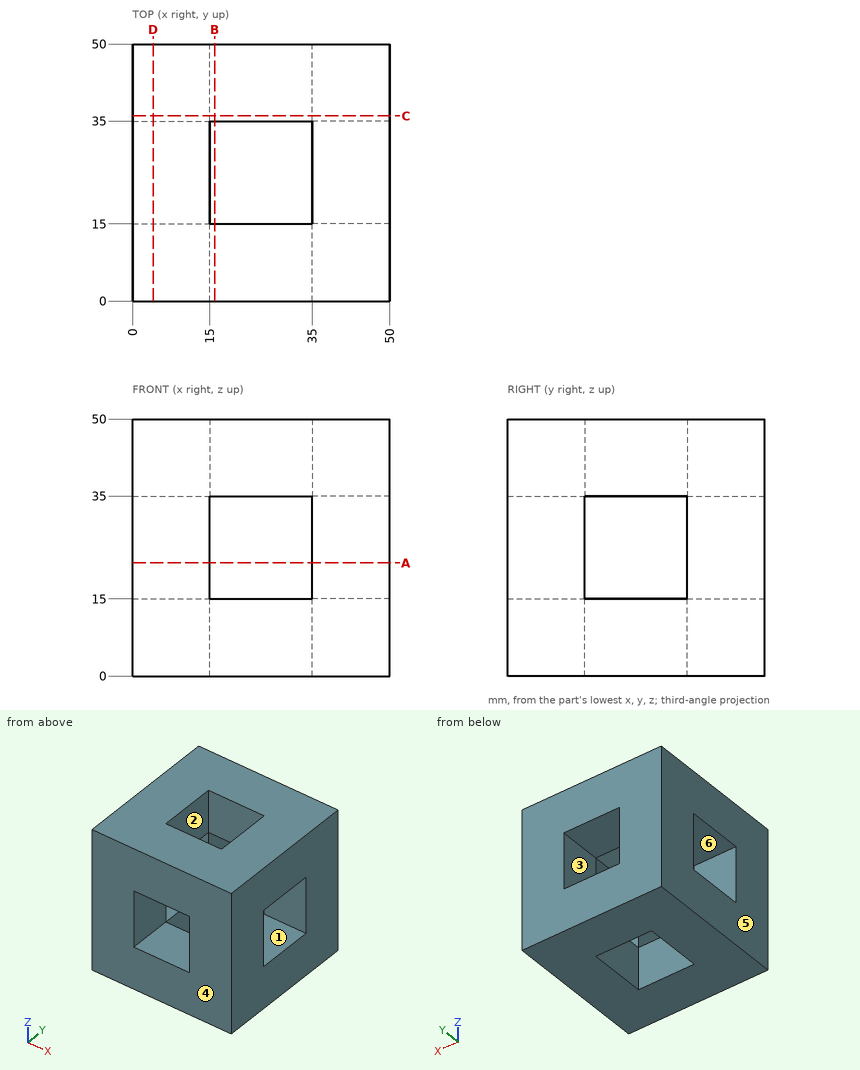
Geometry check sheet. Reference: drawing and pictorial views, mm from the part's lowest x, y, z. A direction names the side the tool comes from. Coordinates: 2 decimals unless noted, no trailing zeros. Write each loop counter-clockwise with the first axis right and the second up, starting at its lowest first coordinate (ties: lowest second). Pieces come first, ordered by that corner, then holes. Notation, with made-up numbers: M -27,-35 L 19,-35 A35 cw 19,-2 Z; hole C -12.5,-21.75 d6. An arc over 180 degrees is marked long. Write item = value, one per line. Start each with the question number.
1. Thickness scan on probe 1 along Z at (x, y) = (24, 3.5). Record the ranges inside material, lowest first.
2. Mould release check, pull along Y, two halves, no side actions. Record for the marked faces 4, 5 and 6: pulls with the +Y half, pulls with the -Y half, needs draft (parallel to the pull), parting line crosses it, or undercut.
3. Tool access check on the marked faces 1, 2 and 3. Record the directions out of +Z, -Z, +X, -X, +Y, -Y that give a thin tool (end or side, any length) a straight path to the whole face; none if there is none.
4. Sectioned sample at C-C (y = 36). Record the cut outline in (x, z), then the cut area to 3 significant figures.
5. Sectioned sample at A-A (z = 22). Record the cut outline in (x, y), then the cut area to 3 significant figures.
The answers:
q1.probe_1 = 0 to 15, 35 to 50
q2.face_4 = pulls with the -Y half
q2.face_5 = needs draft
q2.face_6 = undercut
q3.face_1 = +X, -X
q3.face_2 = +Z, -Z
q3.face_3 = +Y, -Y
q4.outline = M 0,0 L 50,0 L 50,50 L 0,50 Z; hole M 15,15 L 35,15 L 35,35 L 15,35 Z
q4.area = 2,100 mm²
q5.outline = M 0,0 L 15,0 L 15,15 L 0,15 Z; M 0,35 L 15,35 L 15,50 L 0,50 Z; M 35,0 L 50,0 L 50,15 L 35,15 Z; M 35,35 L 50,35 L 50,50 L 35,50 Z
q5.area = 900 mm²
